Could you check a few things on this drawing? It's one solid part, dimensions in mm from its lowest x, y, z. A direction names the side the tool comes from. Give positions to 0.01 mm unless a question says otherwise; leave off trailing zeros. Write each loop counter-clockwise with the first axis right and the second up, starting at its lowest first coordinate (ties: lowest second). Pieces come first, ordered by that corner, then holes. Notation, with made-up numbers: (-2.75, 28.5) - (31.25, 28.5) arc R29 cw to (31.25, 60.5) - close; hole circle Ø7 at (80.5, 34). An arc over 180 degrees is marked (long way). One line per item, written item: value. Start each with the question number.
1) Imagine slicing it at A-A on z = 9.5. Write out the boundary of the cut face in (x, y), plus the area to 3 significant figures.
2) Imagine slicing it at C-C on y = 5.9. Write out the boundary of the cut face in (x, z), plus the area to 3 significant figures.
3) We'd pull the mould along Z, two halves only. Please class the marked faces 5, 6 and 7: +Z half, -Z half, draft (parallel to the pull), parting line (faces both ways), or undercut.
4) I'm going to push flat-ended pins straight in: P1, Ø5, axis at x = 16.5, y = 3, coming from the -Z side; P2, Ø5, axis at x = 5, z = 10, coming from the -Y side; P3, Ø5, axis at y = 5.5, z = 12.5, coming from the +X side. Where does each tip first touch, or does it pass through?
5) Imagine slicing it at D-D on z = 5.75. Write out the boundary of the cut face in (x, y).
6) Imagine slicing it at B-B on x = 5. Write out the boundary of the cut face in (y, z), plus the area to 3 significant figures.
7) On a 3-axis mill with a long thin cutter (end or side, diameter ignored), from which of +Z, -Z, +X, -X, +Y, -Y can I reach the whole of each face in a straight line? I mean the marked faces 1, 2, 3 and 4. Say none if no direction works.
8) Please list where these lines run through material, in increasing order: L1, parallel to X at y = 13.5, z = 9; L2, parallel to Z at x = 5, y = 12.7; L3, parallel to Y at x = 15, z = 9.5. Write a range as [from, to].
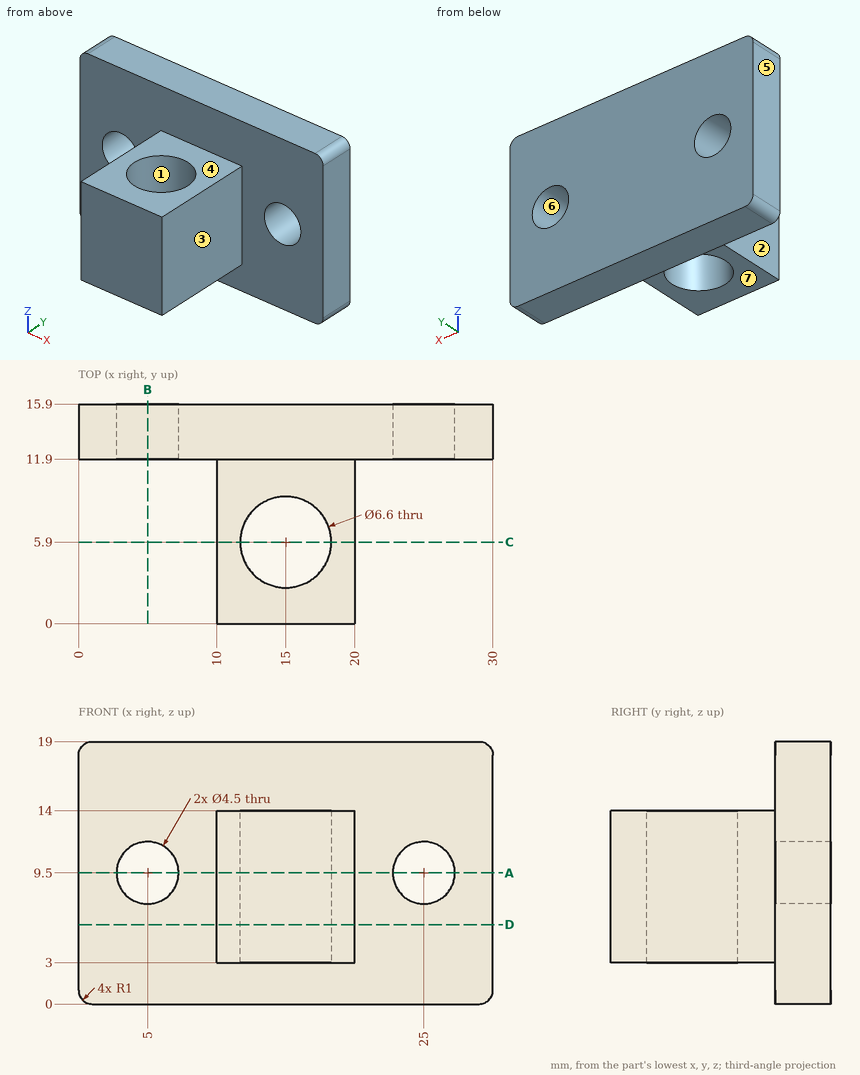
Numbers:
1. outline: (0, 11.9) - (2.75, 11.9) - (2.75, 15.9) - (0, 15.9) - close; (7.25, 11.9) - (10, 11.9) - (10, 0) - (20, 0) - (20, 11.9) - (22.75, 11.9) - (22.75, 15.9) - (7.25, 15.9) - close; (27.25, 11.9) - (30, 11.9) - (30, 15.9) - (27.25, 15.9) - close; hole circle Ø6.6 at (15, 5.9)
1. area: 169 mm^2
2. outline: (10, 3) - (11.7, 3) - (11.7, 14) - (10, 14) - close; (18.3, 3) - (20, 3) - (20, 14) - (18.3, 14) - close
2. area: 37.4 mm^2
3. face 5: draft
3. face 6: undercut
3. face 7: -Z half
4. P1: z = 3
4. P2: y = 11.9
4. P3: x = 20
5. outline: (0, 11.9) - (10, 11.9) - (10, 0) - (20, 0) - (20, 11.9) - (30, 11.9) - (30, 15.9) - (0, 15.9) - close; hole circle Ø6.6 at (15, 5.9)
6. outline: (11.9, 0) - (15.9, 0) - (15.9, 7.25) - (11.9, 7.25) - close; (11.9, 11.75) - (15.9, 11.75) - (15.9, 19) - (11.9, 19) - close
6. area: 58.0 mm^2
7. face 1: +Z, -Z
7. face 2: +Z, -Z, -X, -Y
7. face 3: +Z, -Z, +X, -Y
7. face 4: +Z, +X, -X, -Y
8. L1: [0, 2.81], [7.19, 22.81], [27.19, 30]
8. L2: [0, 7.25], [11.75, 19]
8. L3: [0, 2.6], [9.2, 15.9]
